Geometry check sheet. Reference: drawing and pictorial views, mm from the part's lowest x, y, z. A direction names the side the tool comes from. Round coordinates to 2 decimals unless told otherwise and drop trailing zeros. Order: outer loops, then holes, each group sorted by start corner. A loop starts at its lowest first (then second) coordinate and runs counter-clockwise, first axis right, second up.
(1) Tool access check on the marked faces 1, 2, 3 and 4. Record the directions out of +Z, -Z, +X, -X, +Y, -Y that give a thin tool (end or side, any length) a straight path to the whole face; none if there is none.
(2) Sectioned sample at D-D, the plane x = 22. Enter the section's corners in (y, z).
(3) Sectioned sample at C-C, the plane z = 17.5. Enter the section's corners in (x, y), and give its area (3 significant figures).
(4) Sectioned sample at A-A, the plane y = 70. Enter the section's corners in (x, z), and give its area (3 significant figures).
(5) Sectioned sample at B-B, the plane x = 6.25. Enter the section's corners in (y, z), and give its area (3 significant figures).
(6) Depth check by flat-ended pin: pin 1 (5 mm diameter, centred on x = 12, y = 33, fed in from -Z); pin 2 (4 mm diameter, centred on x = 17.5, z = 6, fed in from -Y); pin 3 (5 mm diameter, centred on x = 10, y = 23.5, fed in from +Z); pin 4 (3.5 mm diameter, centred on x = 12, y = 13, fed in from -Z). Enter the tip coordinate at first touch or a pass-through.
(7) Thickness scan on probe 1 along Z at (x, y) = (22, 7); probe 2 along Y at (x, z) = (2.5, 23); probe 3 along Y at (x, z) = (9.5, 26). Record the ranges inside material, lowest first.
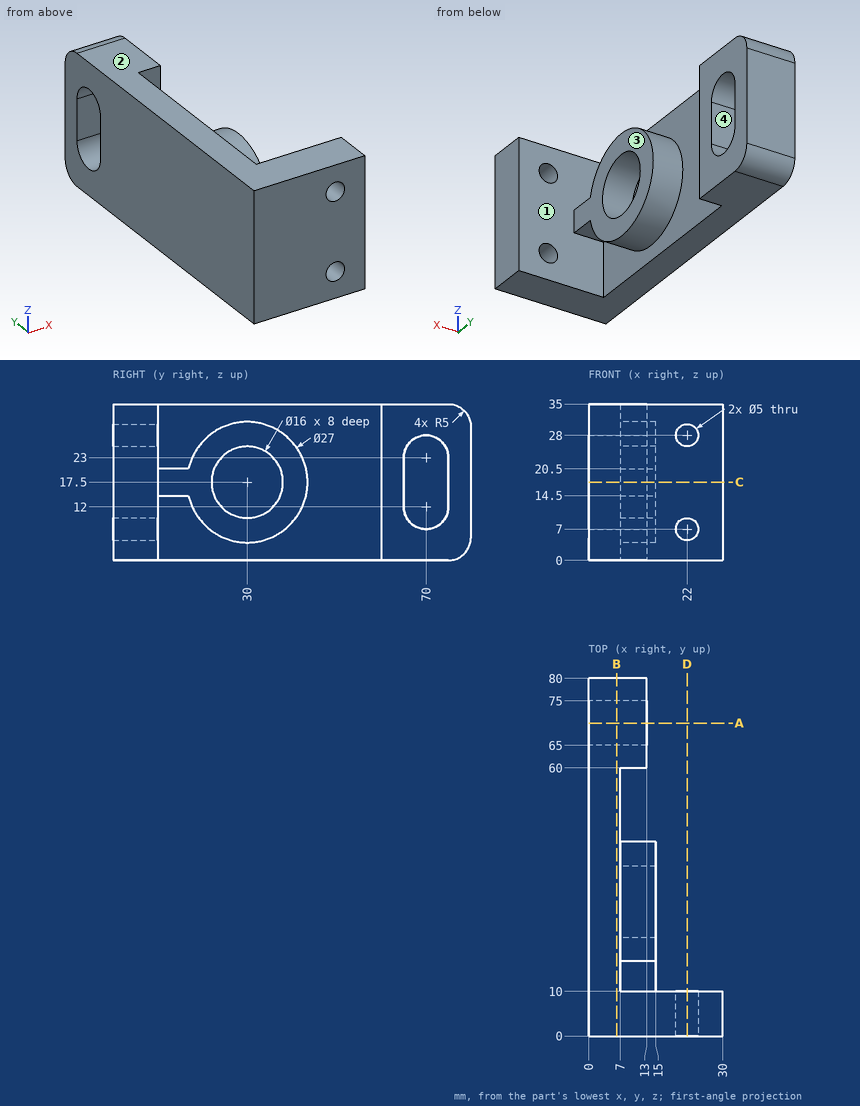
Derived:
1. face 1: +X
1. face 2: +Z, +X, -X, +Y, -Y
1. face 3: +Z, -Z, +X, +Y
1. face 4: +X, -X
2. outline: (0, 0) - (10, 0) - (10, 4.5) - (0, 4.5) - close; (0, 9.5) - (10, 9.5) - (10, 25.5) - (0, 25.5) - close; (0, 30.5) - (10, 30.5) - (10, 35) - (0, 35) - close
3. outline: (0, 0) - (30, 0) - (30, 10) - (15, 10) - (15, 22) - (7, 22) - (7, 38) - (15, 38) - (15, 43.5) - (7, 43.5) - (7, 60) - (13, 60) - (13, 65) - (0, 65) - close; (0, 75) - (13, 75) - (13, 80) - (0, 80) - close
3. area: 920 mm2
4. outline: (0, 0) - (13, 0) - (13, 7) - (0, 7) - close; (0, 28) - (13, 28) - (13, 35) - (0, 35) - close
4. area: 182 mm2
5. outline: (0, 0) - (75, 0) arc R5 ccw to (80, 5) - (80, 30) arc R5 ccw to (75, 35) - (0, 35) - close; hole (65, 12) arc R5 ccw to (75, 12) - (75, 23) arc R5 ccw to (65, 23) - close
5. area: 2,600 mm2
6. pin 1: stops at z = 4.01
6. pin 2: stops at y = 0
6. pin 3: stops at z = 30.39
6. pin 4: stops at z = 14.5
7. probe 1: z = 0 to 4.5, 9.5 to 25.5, 30.5 to 35
7. probe 2: y = 0 to 65, 75 to 80
7. probe 3: y = 0 to 10, 19.51 to 40.49, 60 to 66, 74 to 80
